Here's how the part is built. I have some questions about the finished solid (model axes, mm). A direction names the side the tool comes from. Give positions to 0.01 mm unless a question says otherwise; leave off trailing zeros. Loops run counter-clockwise (first coordinate to the right, second up) from the corner with the lowest first, then second, coordinate; pieces in that order, holes last. Notation, with made-up numbers: (45.25, 24) - (61.25, 24) arc R35 cw to (61.25, 61) - close; hole circle Ø8 at (-4.75, -8). An arc over 180 degrees is marked (long way). Use a Markdown table: item, result.
Autodesk Inventor part; units mm, degrees
ref_plane "YZ Plane" through (0, 0, 0) normal (1, 0, 0) x (0, 1, 0)
ref_plane "XZ Plane" through (0, 0, 0) normal (0, 1, 0) x (-1, 0, 0)
ref_plane "XY Plane" through (0, 0, 0) normal (0, 0, 1) x (1, 0, 0)
sketch "Эскиз1" plane through (0, 0, 0) normal (0, 1, 0) x (-1, 0, 0)
  line L0 (-2.5, 24) -> (2.5, 24)
  line L1 (2.5, 24) -> (2.5, -24)
  line L2 (2.5, -24) -> (-2.5, -24)
  line L3 (-2.5, -24) -> (-2.5, 24)
  line L4 (-2.5, 29) -> (2.5, 29)
  line L5 (2.5, 29) -> (2.5, -29)
  line L6 (2.5, -29) -> (-2.5, -29)
  line L7 (-2.5, -29) -> (-2.5, 29)
  line L8 (2.5, 29) -> (5.5, 29)
  line L9 (5.5, 29) -> (5.5, 19)
  line L10 (5.5, 19) -> (2.5, 19)
  line L11 (2.5, 19) -> (2.5, 29)
  line L12 (-2.5, 19) -> (-5.5, 19)
  line L13 (-5.5, 19) -> (-5.5, 29)
  line L14 (-5.5, 29) -> (-2.5, 29)
  line L15 (-2.5, 29) -> (-2.5, 19)
  line L16 (2.5, -29) -> (5.5, -29)
  line L17 (5.5, -29) -> (5.5, -19)
  line L18 (5.5, -19) -> (2.5, -19)
  line L19 (2.5, -19) -> (2.5, -29)
  line L20 (-2.5, -29) -> (-5.5, -29)
  line L21 (-5.5, -29) -> (-5.5, -19)
  line L22 (-5.5, -19) -> (-2.5, -19)
  line L23 (-2.5, -19) -> (-2.5, -29)
  point P0 (0, 0)
  dimension "d3" = 3
  dimension "d4" = 10
  dimension "d5" = 3
  dimension "d6" = 10
  dimension "d7" = 3
  dimension "d8" = 10
  dimension "d9" = 3
  dimension "d10" = 10
extrude "Выдавливание1" add sketch "Эскиз1" along normal blind 20 contours L0 L1 L2 L3 | L3 L12 L13 L14 L7 | L5 L8 L9 L10 L1 | L3 L7 L20 L21 L22 | L18 L17 L16 L5 L1
sketch "Эскиз2" plane through (2.5, 0, 19) normal (1, 0, 0) x (0, 0, -1)
  line L0 (19, 0) -> (19, 20)
  line L1 (0, 20) -> (38, 20)
  circle A0 centre (19, 10) radius 2
  dimension "d13" = 4
extrude "Выдавливание2" cut sketch "Эскиз2" against normal blind 35
chamfer "Фаска1" distance 2 angle 45 7 edges at (-4, 20, -19) (-4, 0, -19) (4, 20, -19) (4, 20, 19) (-4, 20, 19) (-4, 0, 19) (4, 0, 19)
sketch "Эскиз3" plane through (2.5, 0, -19) normal (1, 0, 0) x (0, 0, -1)
  circle A0 centre (-19, 10) radius 2
  line L0 (-19, 10) -> (-9, 10)
  line L1 (-19, 10) -> (-29, 10)
  circle A1 centre (-29, 10) radius 1.95
  circle A2 centre (-9, 10) radius 1.95
  point P0 (-19, 0)
  dimension "d19" = 10
  dimension "d20" = 10
  dimension "d21" = 3.9
  dimension "d22" = 3.9
extrude "Выдавливание3" cut sketch "Эскиз3" against normal blind 22 contours A1 | A2
properties part number "МД.001.1003 - Каретка" material "Пластик АБС"
(1) Suppose I cut it at D-D on y = 14.75. Write out the boundary of the cut face in (x, z).
A:
| item | result |
|---|---|
| outline | (-5.5, -29) - (-2.5, -29) - (-2.5, -24) - (2.5, -24) - (2.5, -29) - (5.5, -29) - (5.5, -19) - (2.5, -19) - (2.5, 19) - (5.5, 19) - (5.5, 29) - (2.5, 29) - (2.5, 24) - (-2.5, 24) - (-2.5, 29) - (-5.5, 29) - (-5.5, 19) - (-2.5, 19) - (-2.5, -19) - (-5.5, -19) - close |
(2) Will these pins go through, and if not, where does the flat tip stop? pin 1 (10 mm diameter, centred on y = 12, z = -3.5, fed in from +X); pin 2 (12 mm diameter, centred on y = 4, z = -7.5, fed in from -X); pin 3 (1 mm diameter, centred on x = 0.5, y = 14.5, fed in from +Z).
A:
| item | result |
|---|---|
| pin 1 | x = 2.5 |
| pin 2 | x = -2.5 |
| pin 3 | z = 24 |
(3) On a 3-axis mill with a long thin cutter (end or side, diameter ignored), from which of +Z, -Z, +X, -X, +Y, -Y can I reach the whole of each face in a straight line? I mean faces 1 (the face through (-4, 19, 20)), 2 (the face through (-4, 10, 19)), 3 (the face through (-4, 1, -20)), 4 (the face through (4, 9, -19)), 5 (the face through (2.5, 10, 26)). Say none if no direction works.
A:
| item | result |
|---|---|
| face 1 | -X, +Y |
| face 2 | -X, +Y, -Y |
| face 3 | -X, -Y |
| face 4 | +X, +Y, -Y |
| face 5 | +Z, +Y, -Y |
(4) Suppose I cut it at B-B on y = 10. Count the separate pieces of the cut face and the enclosed holes in it, plus the area to 3 significant figures.
A:
| item | result |
|---|---|
| separate pieces | 4 |
| enclosed holes | 0 |
| area | 301 mm2 |
(5) If I drill on line 1 (Z direction, x = -3, y = 7.75); line 2 (X direction, y = 2, z = 24.5); line 3 (Y direction, x = 0.2, z = 10), over which ranges is the centre line in solid material (lowest first)?
A:
| item | result |
|---|---|
| line 1 | -29 to -19, 19 to 29 |
| line 2 | -5.5 to -2.5, 2.5 to 5.5 |
| line 3 | 0 to 8.05, 11.95 to 20 |
(6) Suppose I cut it at A-A on z = -10. Write out the boundary of the cut face in (x, y), plus the area to 3 significant figures.
A:
| item | result |
|---|---|
| outline | (-2.5, 0) - (2.5, 0) - (2.5, 8.05) - (-2.5, 8.05) - close; (-2.5, 11.95) - (2.5, 11.95) - (2.5, 20) - (-2.5, 20) - close |
| area | 80.5 mm2 |
(7) Suppose I cut it at C-C on x = 1. Write out the boundary of the cut face in (y, z).
A:
| item | result |
|---|---|
| outline | (0, -24) - (20, -24) - (20, 24) - (0, 24) - close; hole circle Ø4 at (10, 0); hole circle Ø3.9 at (10, -10); hole circle Ø3.9 at (10, 10) |
(8) We'd pull the mould along Y, two halves only. Please class faces 6 (the face through (0.04, 8.27, 9.1)), 7 (the face through (4, 1, 20)), 8 (the face through (5.5, 10, -24)): pulls with the +Y half, pulls with the -Y half, needs draft (parallel to the pull), parting line crosses it, or undercut.
A:
| item | result |
|---|---|
| face 6 | undercut |
| face 7 | pulls with the -Y half |
| face 8 | needs draft |
